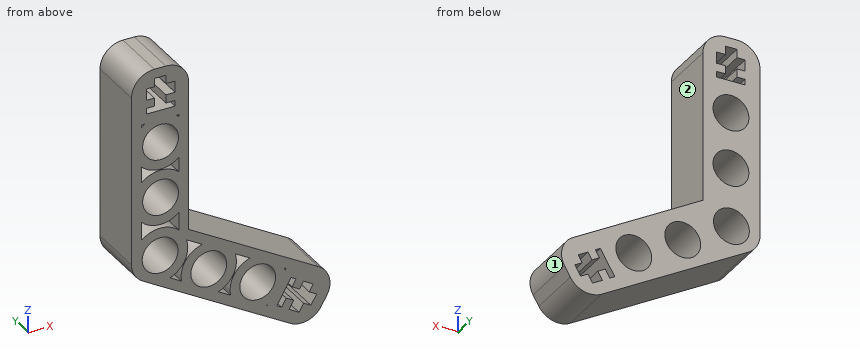
from build123d import *

# Parameters (mm, degrees)
F0_R        = 4.7450397895
F0_R_2      = 3.9830397895
F1_DEPTH    = 12.7
F2_R        = 5.08
F3_R        = 5.08
F4_R        = 5.08
F5_R        = 5.08
F6_R        = 5.08
F7_T        = 2.159
F7_T3_DEPTH = 17.018


# Not quite as in the source:
# - a shell that OpenCascade refuses in one call is made with other operations: the cavity is built on its own and cut out


with BuildPart() as f1:
    # F0 (on Front) → F1 (new body)
    with BuildSketch(Plane.XZ):
        Polygon((-41.5410360719, 38.3876515813), (-54.2410360719, 38.3876515813), (-54.2410360719, -7.3323484187), (-14.6463546109, -30.1923484187), (-8.2963546109, -19.1938257906), (-41.5410360719, 0), align=None)
        with Locations((-47.8910360719, -4.0453961561)):
            Circle(F0_R, mode=Mode.SUBTRACT)
        with Locations((-37.0812863111, -10.2078355849)):
            Circle(F0_R, mode=Mode.SUBTRACT)
        with Locations((-26.2024924159, -16.2752047181)):
            Circle(F0_R, mode=Mode.SUBTRACT)
        Polygon((-16.936610418, -20.4973731492), (-16.0464954671, -18.9635408218), (-13.8496222672, -20.238432246), (-14.7397372181, -21.7722645735), (-13.1120789848, -22.7168286582), (-14.386970409, -24.9137018581), (-16.0146286424, -23.9691377734), (-17.0368508278, -25.7306152458), (-19.2337240277, -24.4557238215), (-18.2115018423, -22.6942463491), (-19.8636214544, -21.7354868152), (-20.8795533344, -23.4861249306), (-21.9779899344, -22.8486792184), (-18.7907613738, -17.3564962187), (-17.6923247738, -17.9939419308), (-18.5887300301, -19.5386136153), align=None, mode=Mode.SUBTRACT)
        with Locations((-47.7926284075, 9.0494407341)):
            Circle(F0_R, mode=Mode.SUBTRACT)
        with Locations((-47.7926284075, 21.5367097408)):
            Circle(F0_R, mode=Mode.SUBTRACT)
        Polygon((-49.1420680823, 31.8705764772), (-50.9154633185, 31.8745224733), (-50.909811558, 34.4145161854), (-49.1364163218, 34.4105701893), (-49.1322289456, 36.2924456105), (-46.5922352335, 36.2867938499), (-46.5964226097, 34.4049184288), (-44.5598272777, 34.4003867841), (-44.5654790382, 31.860393072), (-46.6020743702, 31.8649247167), (-46.6061752529, 30.0219208878), (-44.5537036309, 30.0173539166), (-44.5565518125, 28.7373345026), (-50.9065360928, 28.7514639039), (-50.9036879112, 30.0314833179), (-49.146168965, 30.0275726483), align=None, mode=Mode.SUBTRACT)
        with Locations((-47.7926284075, 21.5367097408)):
            Circle(F0_R)
        with Locations((-47.7926284075, 21.5367097408)):
            Circle(F0_R_2, mode=Mode.SUBTRACT)
        with Locations((-47.7926284075, 9.0494407341)):
            Circle(F0_R)
        with Locations((-47.7926284075, 9.0494407341)):
            Circle(F0_R_2, mode=Mode.SUBTRACT)
        with Locations((-47.8910360719, -4.0453961561)):
            Circle(F0_R)
        with Locations((-47.8910360719, -4.0453961561)):
            Circle(F0_R_2, mode=Mode.SUBTRACT)
        with Locations((-37.0812863111, -10.2078355849)):
            Circle(F0_R)
        with Locations((-37.0812863111, -10.2078355849)):
            Circle(F0_R_2, mode=Mode.SUBTRACT)
        with Locations((-26.2024924159, -16.2752047181)):
            Circle(F0_R)
        with Locations((-26.2024924159, -16.2752047181)):
            Circle(F0_R_2, mode=Mode.SUBTRACT)
    extrude(amount=F1_DEPTH)

    # F2
    f2_edges = [f1.edges().sort_by_distance(p)[0] for p in [
        (-8.296355, -6.35, -19.193826),
    ]]
    fillet(f2_edges, radius=F2_R)

    # F3
    f3_edges = [f1.edges().sort_by_distance(p)[0] for p in [
        (-14.646355, -6.35, -30.192348),
    ]]
    fillet(f3_edges, radius=F3_R)

    # F4
    f4_edges = [f1.edges().sort_by_distance(p)[0] for p in [
        (-54.241036, -6.35, 38.387652),
    ]]
    fillet(f4_edges, radius=F4_R)

    # F5
    f5_edges = [f1.edges().sort_by_distance(p)[0] for p in [
        (-41.541036, -6.35, 38.387652),
    ]]
    fillet(f5_edges, radius=F5_R)

    # F6
    f6_edges = [f1.edges().sort_by_distance(p)[0] for p in [
        (-54.241036, -6.35, -7.332348),
    ]]
    fillet(f6_edges, radius=F6_R)

    # F7: shell of thickness 2.159, made by hand


with BuildPart() as f7_core1:
    # F7_t2: copy of F1
    add(f1.part)

    # the walls: a layer under each face that stays
    f7_faces = [f7_core1.faces().sort_by_distance(p)[0] for p in [
        (-46.8934906703, 0, 5.0273561069),
        (-54.2410360719, -6.35, 14.454121265),
        (-53.5604451231, -6.35, -6.9394090512),
        (-52.7531385203, -6.35, 36.8997540297),
        (-35.373399867, -6.35, -18.2255832606),
        (-47.8910360719, -6.35, 38.3876515813),
        (-15.190962913, -6.35, -28.159842565),
        (-43.0289336235, -6.35, 36.8997540297),
        (-11.4713546109, -6.35, -24.6930871047),
        (-41.5410360719, -6.35, 16.6538257906),
        (-10.3288604645, -6.35, -19.7384340928),
        (-27.118399867, -6.35, -8.3269128953),
        (-51.775668197, -6.35, 21.5367097408),
        (-20.3843756541, -6.35, -20.1025877186),
        (-18.2415430738, -6.35, -17.6752190748),
        (-18.140527402, -6.35, -18.7662777731),
        (-17.7626702241, -6.35, -20.0179933823),
        (-16.4915529426, -6.35, -19.7304569855),
        (-14.9480588672, -6.35, -19.6009865339),
        (-14.2946797427, -6.35, -21.0053484098),
        (-13.9259081015, -6.35, -22.2445466159),
        (-13.7495246969, -6.35, -23.8152652582),
        (-15.2007995257, -6.35, -24.4414198157),
        (-16.5257397351, -6.35, -24.8498765096),
        (-18.1352874278, -6.35, -25.0931695336),
        (-18.722612935, -6.35, -23.5749850853),
        (-19.0375616483, -6.35, -22.2148665822),
        (-20.3715873944, -6.35, -22.6108058729),
        (-21.4287716344, -6.35, -23.1674020745),
        (-46.6041248116, -6.35, 30.9434228022),
        (-45.5799394419, -6.35, 30.0196374022),
        (-44.5551277217, -6.35, 29.3773442096),
        (-47.7315439526, -6.35, 28.7443992033),
        (-50.905112002, -6.35, 29.3914736109),
        (-50.0249284381, -6.35, 30.0295279831),
        (-49.1441185237, -6.35, 30.9490745627),
        (-50.0287657004, -6.35, 31.8725494752),
        (-50.9126374382, -6.35, 33.1445193293),
        (-50.0231139399, -6.35, 34.4125431874),
        (-49.1343226337, -6.35, 35.3515078999),
        (-47.8622320896, -6.35, 36.2896197302),
        (-46.5943289216, -6.35, 35.3458561394),
        (-45.5781249437, -6.35, 34.4026526065),
        (-44.562653158, -6.35, 33.130389928),
        (-45.5837767042, -6.35, 31.8626588943),
        (-51.8740758614, -6.35, -4.0453961561),
        (-41.0643261006, -6.35, -10.2078355849),
        (-51.775668197, -6.35, 9.0494407341),
        (-30.1855322054, -6.35, -16.2752047181),
    ]]
    thicken(f7_faces, amount=-F7_T, mode=Mode.SUBTRACT)

    # F7_s4 → F7_t3 (cut)
    with BuildSketch(Plane.XZ.offset(-2.159)):
        Polygon((-41.5086510719, 0.0186974885), (-43.7000360719, 0), (-43.7000360719, -1.2464992312), (-42.6205360719, -1.8697488468), align=None)
        Polygon((-21.9484799351, -22.8408423733), (-23.8453321543, -21.7650215078), (-24.9289898649, -23.6323637277), (-23.061647645, -24.7160214383), align=None)
        Polygon((-18.7829245287, -17.386006218), (-20.6581035937, -16.2728385081), (-19.5744458831, -14.4054962882), (-17.7071036632, -15.4891539988), align=None)
        Polygon((-17.7218347731, -18.0017787759), (-16.6086670632, -16.1265997109), (-14.7413248433, -17.2102574215), (-15.8249825539, -19.0775996414), align=None)
        Polygon((-16.038658622, -18.9930508211), (-17.913837687, -17.8798831112), (-16.8301799764, -16.0125408913), (-14.9628377565, -17.0961986019), align=None)
        Polygon((-13.8791322665, -20.2462690911), (-12.7659645566, -18.3710900261), (-10.8986223367, -19.4547477367), (-11.9822800473, -21.3220899566), align=None)
        Polygon((-13.1415889841, -22.7246655033), (-12.0284212742, -20.8494864383), (-10.1610790543, -21.9331441489), (-11.2447367649, -23.8004863688), align=None)
        Polygon((-14.3948072541, -24.8841918588), (-12.5196281891, -25.9973595687), (-13.6032858997, -27.8647017886), (-15.4706281196, -26.781044078), align=None)
        Polygon((-17.0446876729, -25.7011052464), (-15.1695086079, -26.8142729564), (-16.2531663185, -28.6816151763), (-18.1205085384, -27.5979574657), align=None)
        Polygon((-19.2042140284, -24.4478869764), (-20.3173817383, -26.3230660414), (-22.1847239582, -25.2394083308), (-21.1010662476, -23.3720661109), align=None)
        Polygon((-20.8873901795, -23.4566149313), (-19.0122111145, -24.5697826412), (-20.0958688251, -26.4371248611), (-21.963211045, -25.3534671505), align=None)
        Polygon((-44.5753416174, 29.99581201), (-44.5488996345, 32.1763485719), (-42.3899049792, 32.1715445754), (-42.3947089756, 30.0125499201), align=None)
        Polygon((-44.578093719, 28.7589724891), (-42.3975571572, 28.7325305062), (-42.4023611536, 26.5735358509), (-44.5613558089, 26.5783398473), align=None)
        Polygon((-50.8848981062, 28.7730058105), (-50.9113400892, 26.5924692486), (-53.0703347445, 26.597273245), (-53.0655307481, 28.7562679003), align=None)
        Polygon((-50.8821460046, 30.0098453313), (-53.0626825665, 30.0362873143), (-53.0578785701, 32.1952819696), (-50.8988839148, 32.1904779732), align=None)
        Polygon((-50.893825332, 31.8960643799), (-50.9202673149, 29.715527818), (-53.0792619702, 29.7203318144), (-53.0744579738, 31.8793264697), align=None)
        Polygon((-50.8882696514, 34.3928781989), (-53.0688062133, 34.4193201818), (-53.0640022169, 36.5783148371), (-50.9050075616, 36.5735108407), align=None)
        Polygon((-49.110687039, 36.2708076239), (-51.2912236009, 36.2972496069), (-51.2864196045, 38.4562442622), (-49.1274249492, 38.4514402658), align=None)
        Polygon((-46.61387322, 36.2652519434), (-46.5874312371, 38.4457885052), (-44.4284365818, 38.4409845088), (-44.4332405782, 36.2819898535), align=None)
        Polygon((-44.5814652642, 34.3788448775), (-44.5550232813, 36.5593814394), (-42.396028626, 36.554577443), (-42.4008326224, 34.3955827877), align=None)
        Polygon((-44.5870209448, 31.8820310585), (-42.4064843829, 31.8555890755), (-42.4112883793, 29.6965944202), (-44.5702830346, 29.7013984167), align=None)
    extrude(amount=F7_T3_DEPTH, mode=Mode.SUBTRACT)


with BuildPart() as f1_1:
    add(f1.part)

    # what is left inside the walls is the cavity
    f7_cavity = [f7_core1.part.solids().sort_by_distance(p)[0] for p in [
        (-51.708298, -9.186333, 26.296738),
        (-47.927745, -9.186333, 15.211589),
        (-47.927745, -9.186333, 2.887292),
        (-42.341594, -9.186333, -6.727564),
        (-43.971477, -9.186333, 26.372941),
        (-20.157914, -9.186333, -15.069631),
        (-31.573461, -9.186333, -12.974456),
        (-24.139328, -9.186333, -22.083275),
    ]]
    add(f7_cavity, mode=Mode.SUBTRACT)


solid = f1_1.part
Work out the finished part from the listing and answer in its coordinate system (mm). Face numbers are marked on the shaded views. A direction names the side the tool comes from. Coordinates: 2 decimals unless noted, no trailing zeros. Write each loop counter-clockwise with the first axis right and the second up, starting at its lowest first coordinate (ties: lowest second). Pieces come first, ordered by that corner, then holes. Notation, with made-up numbers: M 1,63 L 53,63 A35 ccw 53,96 Z; hole C -11,-14.75 d6. An arc over 180 degrees is marked long. Answer as CSV lines item,"result". Start each with the question number.
Item 1: A tool of negligible diameter and unlimited length cuts with its end or side. For the marked faces 1 and 2, from which of +Z, -Z, +X, -X, +Y, -Y can it reach the whole face along a straight path? Write none if from no direction.
Item 2: Section B-B on y = -8.5 is taken. Give the number of separate pieces and of enclosed holes in the cut face, and give its area (3 significant figures).
Item 3: Section C-C on z = 19 is taken. Write down the section's boundary in (x, y).
Item 4: Section A-A on z = -3 is taken. Write down the section's boundary in (x, y).
Item 5: Flat-ended cylindrical pins translate along their axes: P1, Ø6.5, axis at x = -26.2, z = -16.28, coming from the +Y side; P2, Ø1.5, axis at y = -3.5, z = -10, coming from the +X side; P3, Ø3.5, axis at y = -9, z = 3.5, coming from the +X side; P4, Ø12, axis at x = -44.5, z = 22, coming from the +Y side. Find the tip coordinate at first contact, or state that the pin passes through.
Item 6: Consider L1, parallel to Z at x = -29.5, y = -2.5; L2, parallel to Z at x = -40.5, y = -11.75; L3, parallel to X at y = -2.75, z = 26.5. Determine where each line is inside the solid, lowest interval first.
Checks:
1,face 1,"+X, +Y, -Y"
1,face 2,"+Z, +X, +Y, -Y"
2,separate pieces,"1"
2,enclosed holes,"15"
2,area,"681 mm²"
3,outline,"M -54.24,-12.7 L -50.86,-12.7 L -50.86,0 L -54.24,0 Z; M -44.72,-12.7 L -41.54,-12.7 L -41.54,0 L -44.72,0 Z"
4,outline,"M -54.24,-12.7 L -51.73,-12.7 L -51.73,0 L -54.24,0 Z; M -44.05,-12.7 L -41.84,-12.7 L -41.84,-2.16 L -40.66,-2.16 L -40.66,-12.7 L -36.34,-12.7 L -36.34,0 L -44.05,0 Z"
5,P1,"passes through"
5,P2,"stops at x = -22.92"
5,P3,"stops at x = -41.54"
5,P4,"stops at y = 0"
6,L1,"z = -21.62 to -18.51, -14.04 to -11.09, -9.44 to -6.95"
6,L2,"z = -15.27 to -12.25, -8.16 to -5.11, -3.09 to -0.6"
6,L3,"x = -54.24 to -52.08, -51.41 to -44.17, -43.7 to -41.54"
